Could you check a few things on this model? Use its own coordinates, in mm. A direction names the side the tool comes from. Round coordinates to 2 decimals unless told otherwise and drop trailing zeros. Order: outer loops, then holes, each group sorted by start corner. A loop starts at its lowest first (then second) coordinate and runs counter-clockwise, first axis right, second up.
```python
from build123d import *

# Parameters (mm, degrees)
SKETCH_1_W          = 15
SKETCH_1_H          = 10
EXTRUDE_1_DEPTH     = 4
SKETCH_2_W          = 2
SKETCH_2_H          = 1
CUT_EXTRUDE_1_DEPTH = 16
SKETCH_3_R          = 1
CUT_EXTRUDE_2_DEPTH = 5


with BuildPart() as part:
    # 草图1 → 凸台-拉伸1 (new body)
    with BuildSketch(Plane.XY):
        Rectangle(SKETCH_1_W, SKETCH_1_H)
    extrude(amount=EXTRUDE_1_DEPTH)

    # 草图2 → 切除-拉伸1 (cut, through all)
    with BuildSketch(Plane(origin=(7.5, 0, 0), x_dir=(0, 0, -1), z_dir=(1, 0, 0))):
        with Locations((-2, 4.5)):
            Rectangle(SKETCH_2_W, SKETCH_2_H)
        with Locations((-2, -4.5)):
            Rectangle(SKETCH_2_W, SKETCH_2_H)
    extrude(amount=-CUT_EXTRUDE_1_DEPTH, mode=Mode.SUBTRACT)

    # 草图3 → 切除-拉伸2 (cut, through all)
    with BuildSketch(Plane.XY.offset(4)):
        Circle(SKETCH_3_R)
    extrude(amount=-CUT_EXTRUDE_2_DEPTH, mode=Mode.SUBTRACT)


solid = part.part
```
Q1. Imagine slicing it at D-D, the plane y = 0. Please give me the cut outline in (x, z).
Q2. For faces 5 (the flat face through (0, 4, 2)), 6 (the flat face through (0, -4, 2)), 7 (the flat face through (-0.1, -5, 0.5)), which set-ups out of +Z, -Z, +X, -X, +Y, -Y let a thin tool reach every point of the face, with its end or its side?
Q3. We'd pull the mould along Z, two halves only. Please class faces 1 (the flat face through (-0.1, 1.2, 4)), 2 (the flat face through (-0.1, 1.2, 0)), 3 (the flat face through (0.1, 4.5, 3)), 4 (the flat face through (-0.1, -5, 3.5)): released by +Z, released by -Z, zero draft, split by the parting line, or undercut.
Q4. Imagine slicing it at B-B, the plane x = 0. Please give me the cut outline in (y, z).
Q5. For P1, Ø0.8, axis at x = -3.5, y = -4.5, coming from the -Z side, with a flat end and sliding along its axis, tell me the tip position at first contact or that it passes through.
Q6. Imagine slicing it at A-A, the plane y = -4.5. Please give me the cut outline in (x, z).
Q7. I need wall thicknesses on L1, parallel to Y at x = 0, z = 1.8; L2, parallel to Z at x = 6, y = -4.25; L3, parallel to X at y = 0.75, z = 3.05. Which ranges of each line are inside material? Lowest first, please.
Q8. Imagine slicing it at C-C, the plane z = 3.8. Please give me the cut outline in (x, y).
Filled in:
1. outline: (-7.5, 0) - (-1, 0) - (-1, 4) - (-7.5, 4) - close; (1, 0) - (7.5, 0) - (7.5, 4) - (1, 4) - close
2. face 5: +X, -X, +Y
2. face 6: +X, -X, -Y
2. face 7: +Z, -Z, +X, -X, -Y
3. face 1: released by +Z
3. face 2: released by -Z
3. face 3: undercut
3. face 4: zero draft
4. outline: (-5, 0) - (-1, 0) - (-1, 4) - (-5, 4) - (-5, 3) - (-4, 3) - (-4, 1) - (-5, 1) - close; (1, 0) - (5, 0) - (5, 1) - (4, 1) - (4, 3) - (5, 3) - (5, 4) - (1, 4) - close
5. P1: stops at z = 0
6. outline: (-7.5, 0) - (7.5, 0) - (7.5, 1) - (-7.5, 1) - close; (-7.5, 3) - (7.5, 3) - (7.5, 4) - (-7.5, 4) - close
7. L1: y = -4 to -1, 1 to 4
7. L2: z = 0 to 1, 3 to 4
7. L3: x = -7.5 to -0.66, 0.66 to 7.5
8. outline: (-7.5, -5) - (7.5, -5) - (7.5, 5) - (-7.5, 5) - close; hole circle Ø2 at (0, 0)
